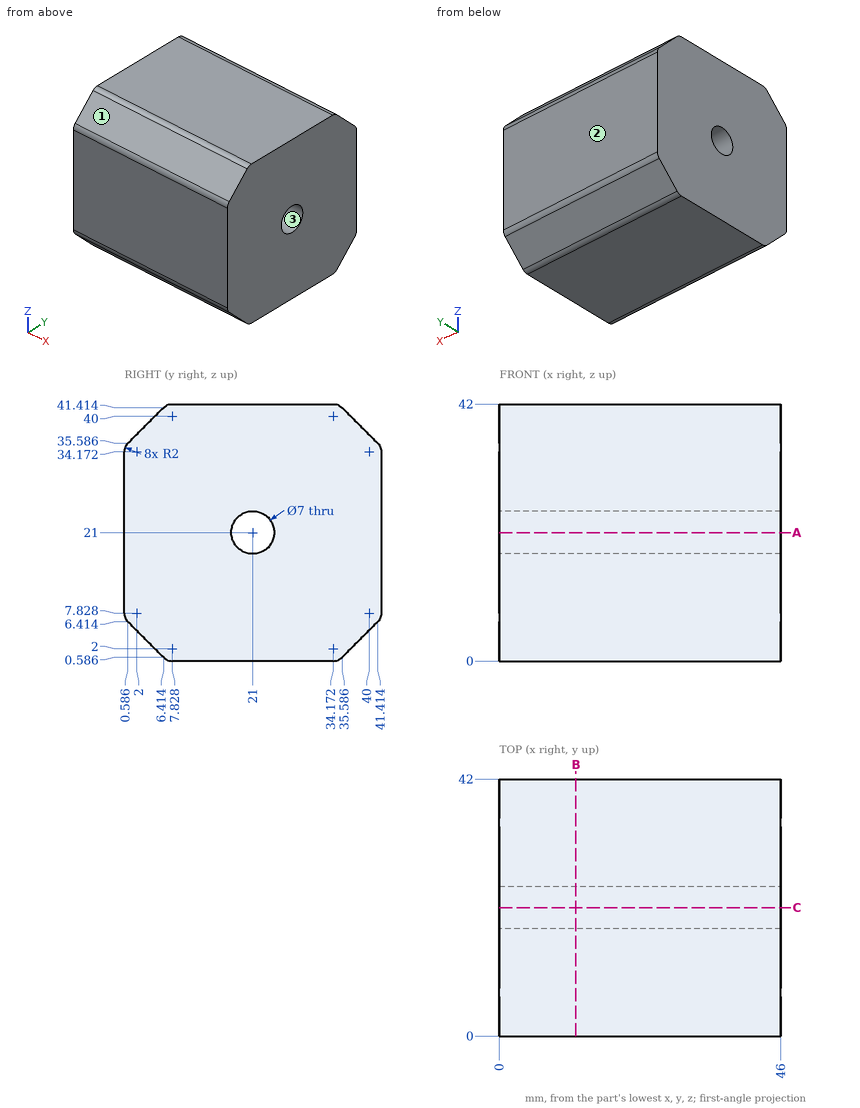
Geometry check sheet. Reference: drawing and pictorial views, mm from the part's lowest x, y, z. Coordinates: 2 decimals unless noted, no trailing zeros. Loops run counter-clockwise (first coordinate to the right, second up) from the corner with the lowest first, then second, coordinate; pieces in that order, holes last. Notation, with made-up numbers: (21.5, -5.75) - (46.5, -5.75) arc R22 ccw to (46.5, 25.25) - close; hole circle Ø11 at (38.5, 89). An arc over 180 degrees is marked (long way). Return JSON: item names as keys, results as strings.
1. Go/stop test with a flat-tipped pin: pin 1 (6 mm diameter, centred on x = 5.5, z = 4.5, fed in from +Y). Record where the tip stops, or that it passes through.
Established:
{"pin 1": "stops at y = 41.97"}
2. Section check A-A, the plane z = 21. Record the boundary of the cut face in (x, y).
Established:
{"outline": "(0, 0) - (46, 0) - (46, 17.5) - (0, 17.5) - close; (0, 24.5) - (46, 24.5) - (46, 42) - (0, 42) - close"}
3. Mould release check, pull along Z, two halves, no side actions. Record for the marked faces 1, 2 and 3: +Z half, -Z half, draft (parallel to the pull), parting line (faces both ways), or undercut.
Established:
{"face 1": "+Z half", "face 2": "draft", "face 3": "undercut"}
4. Thickness scan on L1, parallel to Z at x = 20, y = 21; L2, parallel to Z at x = 18, y = 18.5. Record the ranges inside material, lowest first.
Established:
{"L1": "z = 0 to 17.5, 24.5 to 42", "L2": "z = 0 to 18.55, 23.45 to 42"}
5. Section check B-B, the plane x = 12.5. Record the boundary of the cut face in (y, z) (1 decimal).
Established:
{"outline": "(0, 7.8) arc R2 ccw to (0.6, 6.4) - (6.4, 0.6) arc R2 ccw to (7.8, 0) - (34.2, 0) arc R2 ccw to (35.6, 0.6) - (41.4, 6.4) arc R2 ccw to (42, 7.8) - (42, 34.2) arc R2 ccw to (41.4, 35.6) - (35.6, 41.4) arc R2 ccw to (34.2, 42) - (7.8, 42) arc R2 ccw to (6.4, 41.4) - (0.6, 35.6) arc R2 ccw to (0, 34.2) - close; hole circle Ø7 at (21, 21)"}
